Check sheet for the modelled part. Datum: model origin and axes. Units: mm. A direction names the side the tool comes from. Coordinates: 2 decimals unless noted, no trailing zeros. Loops run counter-clockwise (first coordinate to the right, second up) from the corner with the lowest first, then second, coordinate; pieces in that order, holes last. Notation, with made-up numbers: (74, -34) -> (114, -34) arc R32 ccw to (114, 2) -> close; hole circle Ø8 at (0.25, -29). An arc over 180 degrees is marked (long way). Use one line per item in the form item = value.
from build123d import *

# Parameters (mm, degrees)
BASE_EXTRUDE_DEPTH  = 3.5
SKETCH3_R           = 2.5
BOSS_EXTRUDE1_DEPTH = 16
CHAMFER1_SIZE       = 0.6134
FILLET1_R           = 0.25


with BuildPart() as part:
    # Sketch1 → Base-Extrude (new body)
    with BuildSketch(Plane.XY):
        Polygon((-2.309401077, 4), (2.309401077, 4), (4.618802154, 0), (2.309401077, -4), (-2.309401077, -4), (-4.618802154, 0), align=None)
    extrude(amount=BASE_EXTRUDE_DEPTH)

    # Sketch3 → Boss-Extrude1 (add)
    with BuildSketch(Plane(origin=(0, 0, 0), x_dir=(-1, 0, 0), z_dir=(0, 0, -1))):
        with Locations(Location((0, 0, 0), (0, 0, 180))):
            Circle(SKETCH3_R)
    extrude(amount=BOSS_EXTRUDE1_DEPTH)

    # Chamfer1
    chamfer1_edges = [part.edges().sort_by_distance(p)[0] for p in [
        (-2.5, 0, -16),
    ]]
    chamfer(chamfer1_edges, length=CHAMFER1_SIZE)

    # Fillet1
    fillet1_edges = [part.edges().sort_by_distance(p)[0] for p in [
        (-2.5, 0, 0),
    ]]
    fillet(fillet1_edges, radius=FILLET1_R)


solid = part.part
(1) Section check D-D, the plane x = -3.5. Record the boundary of the cut face in (y, z).
Established:
outline = (-1.94, 0) -> (1.94, 0) -> (1.94, 3.5) -> (-1.94, 3.5) -> close
(2) Section check B-B, the plane z = -0.5. Record the boundary of the cut face in (x, y), plus the area to 3 significant figures.
Established:
outline = circle Ø5 at (0, 0)
area = 19.6 mm²
(3) Go/stop test with flat-tipped pins: P1, Ø1.5, axis at y = 1.5, z = -8, coming from the -X side; P2, Ø3, axis at x = -1.5, z = -6.5, coming from the -Y side; P3, Ø2, axis at y = 2, z = -12, coming from the +X side. Record where each tip stops, or that it passes through.
Established:
P1 = -2.38
P2 = -2.5
P3 = 2.29
(4) Scan lines: line 1 along Z through (x, y) = (2, 2); line 2 along Y through (x, z) = (-1.5, -5.5); line 3 along X through (y, z) = (-0.75, -8.5). Record each from-to range of solid material in increasing order.
Established:
line_1 = 0 to 3.5
line_2 = -2 to 2
line_3 = -2.38 to 2.38
(5) Section check A-A, the plane x = 0. Record the boundary of the cut face in (y, z), plus the area to 3 significant figures.
Established:
outline = (-4, 0) -> (-2.75, 0) arc R0.25 cw to (-2.5, -0.25) -> (-2.5, -15.39) -> (-1.89, -16) -> (1.89, -16) -> (2.5, -15.39) -> (2.5, -0.25) arc R0.25 cw to (2.75, 0) -> (4, 0) -> (4, 3.5) -> (-4, 3.5) -> close
area = 108 mm²
(6) Section check C-C, the plane y = -3. Record the boundary of the cut face in (x, z), plus the area to 3 significant figures.
Established:
outline = (-2.89, 0) -> (2.89, 0) -> (2.89, 3.5) -> (-2.89, 3.5) -> close
area = 20.2 mm²
(7) Tool access check on faces 1 (the cylindrical face through (-2.5, -0.1, -7.7)), 2 (the flat face through (0, 0, -16)). Record the directions out of +Z, -Z, +X, -X, +Y, -Y that give a thin tool (end or side, any length) a straight path to the whole face; none if there is none.
Established:
face_1 = -Z
face_2 = -Z, +X, -X, +Y, -Y
